```python
from build123d import *

# Parameters (mm, degrees)
F0_W     = 76.2
F0_H     = 76.2
F1_DEPTH = 38.1
F2_R     = 25.4
F3_DEPTH = 76.2
F4_R     = 25.4
F5_DEPTH = 76.2
F6_W     = 50.8
F6_H     = 50.8
F7_DEPTH = 76.2


with BuildPart() as f1:
    # F0 (on Front) → F1 (new body, symmetric)
    with BuildSketch(Plane.XZ):
        Rectangle(F0_W, F0_H)
    extrude(amount=F1_DEPTH, both=True)

    # F2 (on face) → F3 (cut, through all)
    with BuildSketch(Plane(origin=(-38.1, 0, 0), x_dir=(0, -1, 0), z_dir=(-1, 0, 0))):
        Circle(F2_R)
    extrude(amount=-F3_DEPTH, mode=Mode.SUBTRACT)

    # F4 (on face) → F5 (cut)
    with BuildSketch(Plane.XZ.offset(38.1)):
        Circle(F4_R)
    extrude(amount=-F5_DEPTH, mode=Mode.SUBTRACT)

    # F6 (on face) → F7 (cut)
    with BuildSketch(Plane.XY.offset(38.1)):
        Rectangle(F6_W, F6_H)
    extrude(amount=-F7_DEPTH, mode=Mode.SUBTRACT)


solid = f1.part
```
Could you check a few things on this model? Use its own coordinates, in mm. A direction names the side the tool comes from. Coordinates: 2 decimals unless noted, no trailing zeros. Order: outer loops, then holes, each group sorted by start corner. A loop starts at its lowest first (then second) coordinate and runs counter-clockwise, first axis right, second up. Notation, with made-up numbers: M 65,83.25 L 82,83.25 A13 ccw 82,97.25 Z; hole C 51.5,50.25 d6. An arc over 180 degrees is marked long. Use a Markdown table: item, result. Add a question column.
Q1. Which directions (+Z, -Z, +X, -X, +Y, -Y) give clear straight access to the entire face, cutting with the end or side of a thin tool? Please do faces 1 (the cylindrical face through (31.661, 5.506, -24.796)), 2 (the flat face through (0, 25.4, -27)).
Q2. If I drill on L1, parallel to X at y = -32, z = 0, over which ranges is the centre line in solid material (lowest first)?
Q3. I want a section at A-A on x = -28. List the corners of the cut face in (y, z) for me.
Q4. I want a section at D-D on x = 0. List the corners of the cut face in (y, z) for me.
Q5. I want a section at C-C on z = 8.5. List the corners of the cut face in (x, y) for me.
Q6. We'd pull the mould along Y, two halves only. Please class faces 3 (the flat face through (-25.4, 0, 28)), 4 (the flat face through (-1, 38.1, 26)), 5 (the flat face through (-26, -1, -38.1)): pulls with the +Y half, pulls with the -Y half, needs draft (parallel to the pull), parting line crosses it, or undercut.
Checked values:
| question | item | result |
|---|---|---|
| 1 | face 1 | +X, -X |
| 1 | face 2 | +Z, -Z |
| 2 | L1 | -38.1 to -25.4, 25.4 to 38.1 |
| 3 | outline | M -38.1,-38.1 L 38.1,-38.1 L 38.1,38.1 L -38.1,38.1 Z; hole C 0,0 d50.8 |
| 4 | outline | M -38.1,-38.1 L -25.4,-38.1 L -25.4,-25.4 L -38.1,-25.4 Z; M -38.1,25.4 L -25.4,25.4 L -25.4,38.1 L -38.1,38.1 Z; M 25.4,-38.1 L 38.1,-38.1 L 38.1,-25.4 L 25.4,-25.4 Z; M 25.4,25.4 L 38.1,25.4 L 38.1,38.1 L 25.4,38.1 Z |
| 5 | outline | M -38.1,-38.1 L -23.94,-38.1 L -23.94,-25.4 L -25.4,-25.4 L -25.4,-23.94 L -38.1,-23.94 Z; M -38.1,23.94 L -25.4,23.94 L -25.4,25.4 L -23.94,25.4 L -23.94,38.1 L -38.1,38.1 Z; M 23.94,-38.1 L 38.1,-38.1 L 38.1,-23.94 L 25.4,-23.94 L 25.4,-25.4 L 23.94,-25.4 Z; M 23.94,25.4 L 25.4,25.4 L 25.4,23.94 L 38.1,23.94 L 38.1,38.1 L 23.94,38.1 Z |
| 6 | face 3 | undercut |
| 6 | face 4 | pulls with the +Y half |
| 6 | face 5 | needs draft |
